Source: CAD feature listing. Evaluate the final solid. Frame: model axes, mm. A direction names the side the tool comes from. Coordinates: 2 decimals unless noted, no trailing zeros. Loops run counter-clockwise (first coordinate to the right, second up) from the corner with the lowest first, then second, coordinate; pieces in that order, holes last.
Item 1: Line query: probe 1 along Z at (x, y) = (-0.5, 4); probe 2 along X at (y, z) = (5.15, -12.5); probe 3 along X at (y, z) = (0.75, 12.5). Output: solid intervals per line, ascending.
Item 2: Section query C-C, the plane x = 1.3. State how many separate pieces and enclosed holes the cut face has, then the cut area to 3 significant figures.
Item 3: Pull-direction query (X, two-part tool) for faces 1 (the flat face through (0, 0, 0)), 2 (the cylindrical face through (0.143, 5.028, -28.247)), 3 (the cylindrical face through (1.32, 3.46, -29.97)); classes: +X half, -X half, draft (parallel to the pull), parting line (faces both ways), or undercut.
Item 4: Section query A-A, the plane z = 0. Return the cut outline in (x, y), then the cut area to 3 significant figures.
Item 5: Reachability of faces 4 (the cylindrical face through (-20.265, 1.479, -14.011)), 5 (the cylindrical face through (-21.508, 5.028, 9.253)) from +Z, -Z, +X, -X, +Y, -Y: full face, straight path, thin tool, end or side. Return the list, or none.
Item 6: Section query D-D, the plane y = 13. Return the cut outline in (x, z), then the cut area to 3 significant figures.
Item 7: Section query B-B, the plane y = 5.5. Return the cut outline in (x, z).
Item 8: Pin query (flat end, axial travel): pin 1 Ø5 at (x, y) = (-2, 13) entering from +Z; pin 2 Ø2 at (y, z) = (17.5, 11.5) entering from +X; pin 3 Ø12 at (x, y) = (-2.5, 13.5) entering from -Z. Return the tip coordinate at first contact, or that it passes through.
```python
from build123d import *

# Parameters (mm, degrees)
SKETCH1_R           = 30
SKETCH1_R_2         = 2.05
BOSS_EXTRUDE1_DEPTH = 7
SKETCH2_R           = 12.5
BOSS_EXTRUDE2_DEPTH = 11
SKETCH3_R           = 10
BOSS_EXTRUDE3_DEPTH = 11
FILLET1_R           = 0.5
SKETCH4_R           = 3.25
CUT_EXTRUDE1_DEPTH  = 4
SKETCH5_R           = 8.5
BOSS_EXTRUDE4_DEPTH = 7


with BuildPart() as part:
    # Sketch1 → Boss-Extrude1 (new body)
    with BuildSketch(Plane(origin=(0, 0, 0), x_dir=(1, 0, 0), z_dir=(0, 1, 0))):
        with Locations(Location((0, 0, 0), (0, 0, 270))):
            Circle(SKETCH1_R)
        with Locations(Location((0, 25, 0), (0, 0, 270))):
            Circle(SKETCH1_R_2, mode=Mode.SUBTRACT)
        with Locations(Location((21.650635095, 12.5, 0), (0, 0, 270))):
            Circle(SKETCH1_R_2, mode=Mode.SUBTRACT)
        with Locations(Location((21.650635095, -12.5, 0), (0, 0, 270))):
            Circle(SKETCH1_R_2, mode=Mode.SUBTRACT)
        with Locations(Location((0, -25, 0), (0, 0, 270))):
            Circle(SKETCH1_R_2, mode=Mode.SUBTRACT)
        with Locations(Location((-21.650635095, -12.5, 0), (0, 0, 270))):
            Circle(SKETCH1_R_2, mode=Mode.SUBTRACT)
        with Locations(Location((-21.650635095, 12.5, 0), (0, 0, 270))):
            Circle(SKETCH1_R_2, mode=Mode.SUBTRACT)
    extrude(amount=BOSS_EXTRUDE1_DEPTH)

    # Sketch2 → Boss-Extrude2 (add)
    with BuildSketch(Plane(origin=(0, 7, 0), x_dir=(1, 0, 0), z_dir=(0, 1, 0))):
        with Locations(Location((-1.3, 0, 0), (0, 0, 270))):
            Circle(SKETCH2_R)
    extrude(amount=BOSS_EXTRUDE2_DEPTH)

    # Sketch3 → Boss-Extrude3 (add)
    with BuildSketch(Plane(origin=(0, 18, 0), x_dir=(1, 0, 0), z_dir=(0, 1, 0))):
        with Locations(Location((1.3, 0, 0), (0, 0, 17.874562015))):
            Circle(SKETCH3_R)
    extrude(amount=BOSS_EXTRUDE3_DEPTH)

    # Fillet1
    # the kernel refuses this fillet: 0.5 mm, written as the material it takes off along each edge
    with BuildSketch(Plane(origin=(0, 0, 0), x_dir=(0, 0, 1), z_dir=(-1, 0, 0))) as fillet1_piece_1:
        with BuildLine():
            CenterArc((30 - FILLET1_R, FILLET1_R), FILLET1_R, 270, 90)
            Line((30 - FILLET1_R, 0), (30, 0))
            Line((30, 0), (30, FILLET1_R))
        make_face()
    revolve(axis=Axis((0, 0, 0), (0, 1, 0)), mode=Mode.SUBTRACT)
    with BuildSketch(Plane(origin=(-1.3, 18, 0), x_dir=(0.9891034712042164, 0, -0.14722202026792702), z_dir=(0.14722202026792702, 0, 0.9891034712042164))) as fillet1_piece_2_section:
        with BuildLine():
            CenterArc((12.5 - FILLET1_R, -FILLET1_R), FILLET1_R, 0, 90)
            Line((12.5 - FILLET1_R, 0), (12.5, 0))
            Line((12.5, 0), (12.5, -FILLET1_R))
        make_face()
    fillet1_piece_2 = revolve(axis=Axis((-1.3, 18, 0), (0, 1, 0)), revolution_arc=261.534027286, mode=Mode.PRIVATE)
    fillet1_piece_2 = fillet1_piece_2 - Plane(origin=(1.3, 17.863633117, 0), x_dir=(0.9517307692321948, 0, -0.3069341018796947), z_dir=(0, -1, 0)) * Cylinder(10, 50, mode=Mode.PRIVATE)
    add(fillet1_piece_2, mode=Mode.SUBTRACT)
    with BuildSketch(Plane(origin=(1.3, 29, 0), x_dir=(0.9517307692321948, 0, -0.3069341018796947), z_dir=(0.3069341018796947, 0, 0.9517307692321948))) as fillet1_piece_3:
        with BuildLine():
            CenterArc((10 - FILLET1_R, -FILLET1_R), FILLET1_R, 0, 90)
            Line((10 - FILLET1_R, 0), (10, 0))
            Line((10, 0), (10, -FILLET1_R))
        make_face()
    revolve(axis=Axis((1.3, 29, 0), (0, 1, 0)), mode=Mode.SUBTRACT)
    with BuildSketch(Plane(origin=(0, 7, 0), x_dir=(0, 0, 1), z_dir=(-1, 0, 0))) as fillet1_piece_4:
        with BuildLine():
            CenterArc((30 - FILLET1_R, -FILLET1_R), FILLET1_R, 0, 90)
            Line((30 - FILLET1_R, 0), (30, 0))
            Line((30, 0), (30, -FILLET1_R))
        make_face()
    revolve(axis=Axis((0, 7, 0), (0, 1, 0)), mode=Mode.SUBTRACT)
    with BuildSketch(Plane(origin=(-1.3, 18, 0), x_dir=(0, 0, 1), z_dir=(-1, 0, 0))) as fillet1_piece_5_section:
        with BuildLine():
            CenterArc((12.5 - FILLET1_R, -FILLET1_R), FILLET1_R, 0, 90)
            Line((12.5 - FILLET1_R, 0), (12.5, 0))
            Line((12.5, 0), (12.5, -FILLET1_R))
        make_face()
    fillet1_piece_5 = revolve(axis=Axis((-1.3, 18, 0), (0, 1, 0)), revolution_arc=81.517031171, mode=Mode.PRIVATE)
    fillet1_piece_5 = fillet1_piece_5 - Plane(origin=(1.3, 17.860140993, 0), x_dir=(0.9517307692321948, 0, -0.3069341018796947), z_dir=(0, -1, 0)) * Cylinder(10, 50, mode=Mode.PRIVATE)
    add(fillet1_piece_5, mode=Mode.SUBTRACT)

    # Sketch4 → Cut-Extrude1 (cut)
    with BuildSketch(Plane(origin=(0, 7, 0), x_dir=(1, 0, 0), z_dir=(0, 1, 0))):
        with Locations(Location((0, 25, 0), (0, 0, 270))):
            Circle(SKETCH4_R)
        with Locations(Location((21.650635095, 12.5, 0), (0, 0, 270))):
            Circle(SKETCH4_R)
        with Locations(Location((21.650635095, -12.5, 0), (0, 0, 270))):
            Circle(SKETCH4_R)
        with Locations(Location((0, -25, 0), (0, 0, 270))):
            Circle(SKETCH4_R)
        with Locations(Location((-21.650635095, -12.5, 0), (0, 0, 270))):
            Circle(SKETCH4_R)
        with Locations(Location((-21.650635095, 12.5, 0), (0, 0, 270))):
            Circle(SKETCH4_R)
    extrude(amount=-CUT_EXTRUDE1_DEPTH, mode=Mode.SUBTRACT)

    # Sketch5 → Boss-Extrude4 (add)
    with BuildSketch(Plane(origin=(0, 29, 0), x_dir=(1, 0, 0), z_dir=(0, 1, 0))):
        with Locations(Location((0, 0, 0), (0, 0, 137.562092195))):
            Circle(SKETCH5_R)
    extrude(amount=BOSS_EXTRUDE4_DEPTH)


solid = part.part
```
Verdict:
1. probe 1: z = -30 to -28.21, -21.79 to 21.79, 28.21 to 30
1. probe 2: x = -27.27 to -24.9, -18.4 to 18.4, 24.9 to 27.27
1. probe 3: x = -27.27 to -23.7, -19.6 to 19.6, 23.7 to 27.27
2. separate pieces: 3
2. enclosed holes: 0
2. area: 959 mm2
3. face 1: draft
3. face 2: undercut
3. face 3: parting line
4. outline: (-30, 0.5) arc R0.5 ccw to (-29.5, 0) - (29.5, 0) arc R0.5 ccw to (30, 0.5) - (30, 6.5) arc R0.5 ccw to (29.5, 7) - (11.2, 7) - (11.2, 18) - (11.3, 18) - (11.3, 28.5) arc R0.5 ccw to (10.8, 29) - (8.5, 29) - (8.5, 36) - (-8.5, 36) - (-8.5, 29) - (-8.2, 29) arc R0.5 ccw to (-8.7, 28.5) - (-8.7, 18) - (-13.3, 18) arc R0.5 ccw to (-13.8, 17.5) - (-13.8, 7) - (-29.5, 7) arc R0.5 ccw to (-30, 6.5) - close
4. area: 1,030 mm2
5. face 4: +Y, -Y
5. face 5: +Y
6. outline: circle Ø25 at (-1.3, 0)
6. area: 491 mm2
7. outline: circle Ø60 at (0, 0); hole circle Ø6.5 at (-21.65, -12.5); hole circle Ø6.5 at (-21.65, 12.5); hole circle Ø6.5 at (0, -25); hole circle Ø6.5 at (0, 25); hole circle Ø6.5 at (21.65, -12.5); hole circle Ø6.5 at (21.65, 12.5)
8. pin 1: stops at z = 12.5
8. pin 2: stops at x = 5.48
8. pin 3: stops at z = -12.5
